Read the model definition and answer for the solid it produces. Units are mm, in the model's axes. Face numbers are marked on the shaded views. A direction names the side the tool comes from. Give positions to 0.01 mm unless a question says otherwise; leave off trailing zeros. Order: outer loops, then holes, each group sorted by start corner. A loop starts at its lowest first (then second) coordinate and runs counter-clockwise, first axis right, second up.
Item 1: Find the intervals of material crossed by line 1 along Y through (x, z) = (-35.5, 3.5); line 2 along Z through (x, y) = (0, 14.75); line 3 along Y through (x, z) = (3, 6), in increasing order.
Item 2: A cutting plane is placed at C-C (y = 13). Write down the section's boundary in (x, z) (3 decimals), plus the area to 3 significant figures.
Item 3: The mould has two halves that part along Z. Classify the marked faces 1 and 2: +Z half, -Z half, draft (parallel to the pull), parting line (faces both ways), or undercut.
Item 4: Given pin 1 Ø5 at (y, z) = (15, 19.5) entering from +X (3 decimals); pin 2 Ø1 at (x, y) = (26, 7.5) entering from +Z; pin 3 Ø4 at (y, z) = (11, -20.5) entering from -X (3 decimals), each flat-ended and moving along its own axis, determine where each tip first touches the part or whether it passes through.
Item 5: A cutting plane is placed at A-A (x = -7). Write down the section's boundary in (y, z).
Item 6: Which of the six approach directions +Z, -Z, +X, -X, +Y, -Y give full straight-line access (tool end or side, diameter ignored) to the marked faces 3 and 4?
Item 7: A cutting plane is placed at B-B (z = 19.5). Write down the section's boundary in (x, y) (3 decimals).
Item 8: A cutting plane is placed at D-D (z = 39). Write down the section's boundary in (x, y) (3 decimals), plus the area to 3 significant figures.
from build123d import *

# Parameters (mm, degrees)
SKETCH1_W           = 85.47
SKETCH1_H           = 143.2
BOSS_EXTRUDE1_DEPTH = 4.92
SKETCH2_W           = 62.81
SKETCH2_H           = 91.76
BOSS_EXTRUDE2_DEPTH = 12.75
SKETCH3_R           = 2.33
BOSS_EXTRUDE3_DEPTH = 14.9


with BuildPart() as part:
    # Sketch1 → Boss-Extrude1 (new body)
    with BuildSketch(Plane(origin=(0, 0, 0), x_dir=(1, 0, 0), z_dir=(0, 1, 0))):
        Rectangle(SKETCH1_W, SKETCH1_H)
    extrude(amount=BOSS_EXTRUDE1_DEPTH)

    # Sketch2 → Boss-Extrude2 (add)
    with BuildSketch(Plane(origin=(0, 4.92, 0), x_dir=(1, 0, 0), z_dir=(0, 1, 0))):
        with Locations((0, 22.2)):
            Rectangle(SKETCH2_W, SKETCH2_H)
    extrude(amount=BOSS_EXTRUDE2_DEPTH)

    # Sketch3 → Boss-Extrude3 (add)
    with BuildSketch(Plane(origin=(0, 4.92, 0), x_dir=(1, 0, 0), z_dir=(0, 1, 0))):
        with Locations((0, -32.53)):
            Circle(SKETCH3_R)
        with Locations((-30.156916038, -60.313935435)):
            Circle(SKETCH3_R)
    extrude(amount=BOSS_EXTRUDE3_DEPTH)


solid = part.part
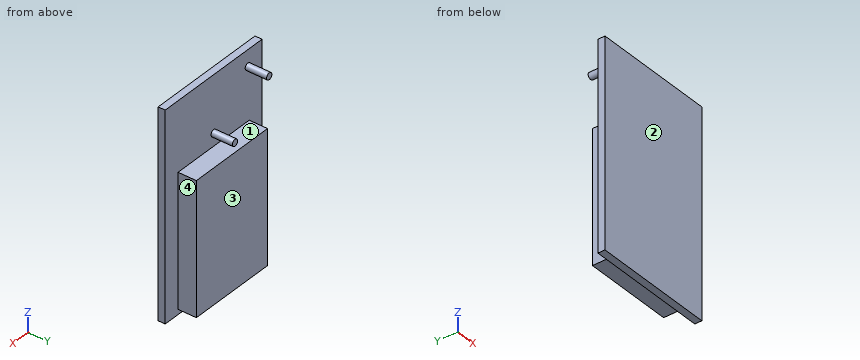
Response values:
1. line 1: y = 0 to 4.92
1. line 2: z = -68.08 to 23.68, 30.2 to 34.86
1. line 3: y = 0 to 17.67
2. outline: circle Ø4.66 at (-30.157, 60.314); (-31.405, -68.08) - (31.405, -68.08) - (31.405, 23.68) - (-31.405, 23.68) - close; circle Ø4.66 at (0, 32.53)
2. area: 5,800 mm2
3. face 1: undercut
3. face 2: draft
4. pin 1: stops at x = 31.405
4. pin 2: stops at z = 23.68
4. pin 3: stops at x = -31.405
5. outline: (0, -71.6) - (4.92, -71.6) - (4.92, -68.08) - (17.67, -68.08) - (17.67, 23.68) - (4.92, 23.68) - (4.92, 71.6) - (0, 71.6) - close
6. face 3: -Z, +X, -X, +Y
6. face 4: +Z, -Z, +X, +Y
7. outline: (-42.735, 0) - (42.735, 0) - (42.735, 4.92) - (31.405, 4.92) - (31.405, 17.67) - (-31.405, 17.67) - (-31.405, 4.92) - (-42.735, 4.92) - close
8. outline: (-42.735, 0) - (42.735, 0) - (42.735, 4.92) - (-42.735, 4.92) - close
8. area: 421 mm2
